The drawing under review shows one solid part. Ordinate dimensions are in mm from its lowest x, y, z. Give positions to 0.01 mm unless a question says otherwise; leave off trailing zeros. Write each loop counter-clockwise with the first axis right and the second up, starting at its lowest first coordinate (ties: lowest second). Pieces come first, ordered by that corner, then holes. Notation, with made-up numbers: (86, 12.25) -> (141, 12.25) arc R13 cw to (141, 26.25) -> close; hole circle Ø2 at (-22, 76.5). An arc over 180 degrees is marked (long way). Put each result on its own line as item: value. Start each with the question number.
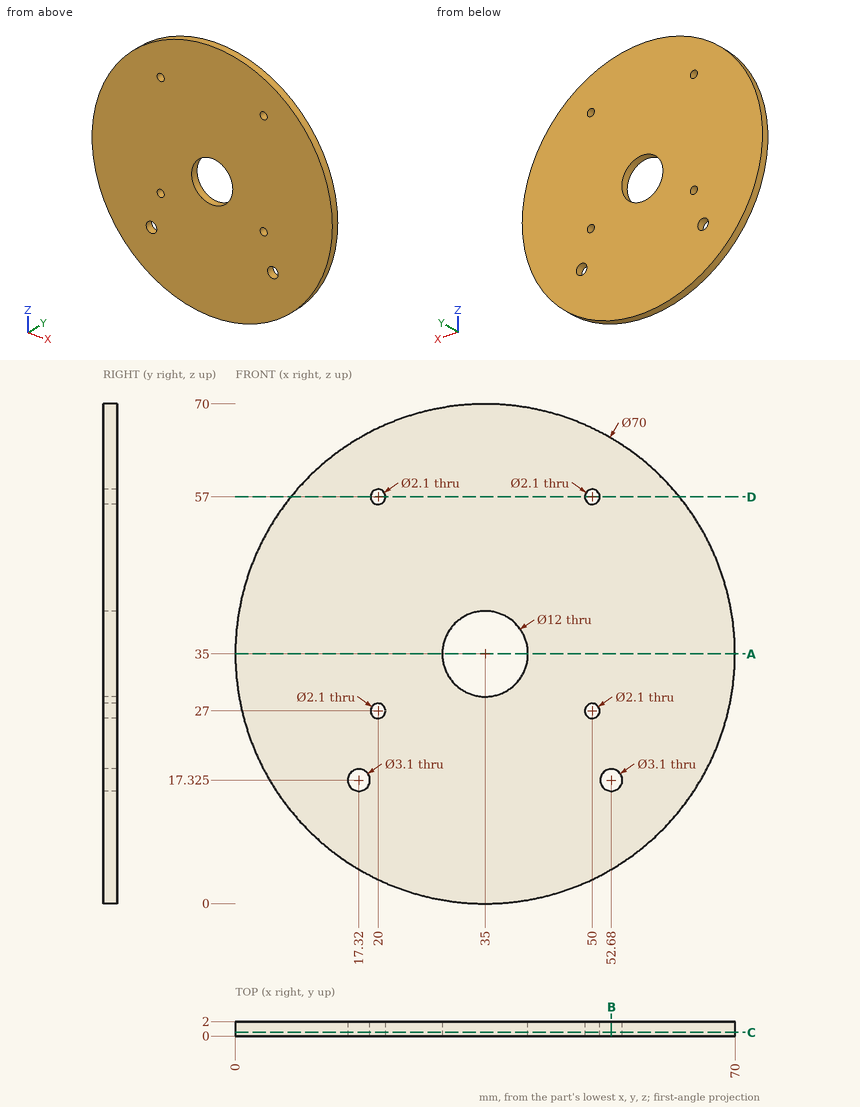
Q1. Take a section at A-A on z = 35. Give the boundary of the cut face in (x, y).
Q2. Take a section at D-D on z = 57. Give the boundary of the cut face in (x, y).
Q3. Take a section at B-B on x = 52.68. Give the boundary of the cut face in (y, z) (1 decimal).
Q4. To check wall thickness, follow probe 1 along Z at (x, y) = (35, 1.2); probe 2 along Z at (x, y) = (50, 1.05); probe 3 along X at (y, z) = (1.6, 30.5). State the ranges of each line that lie inside material, in increasing order. Write a range as from..to.
Q5. For pin 1 (1 mm diameter, centred on y = 1.5, z = 28, fed in from +X); pin 2 (1 mm diameter, centred on x = 34, y = 1.5, fed in from -Z), all flat-tipped, find the tip position at first contact; note any pin that passes through.
Q6. Take a section at C-C on y = 0.5. State how many separate pieces and enclosed holes the cut face has, then the cut area to 3 significant figures.
Result:
1. outline: (0, 0) -> (29, 0) -> (29, 2) -> (0, 2) -> close; (41, 0) -> (70, 0) -> (70, 2) -> (41, 2) -> close
2. outline: (7.78, 0) -> (18.95, 0) -> (18.95, 2) -> (7.78, 2) -> close; (21.05, 0) -> (48.95, 0) -> (48.95, 2) -> (21.05, 2) -> close; (51.05, 0) -> (62.22, 0) -> (62.22, 2) -> (51.05, 2) -> close
3. outline: (0, 4.8) -> (2, 4.8) -> (2, 15.8) -> (0, 15.8) -> close; (0, 18.9) -> (2, 18.9) -> (2, 65.2) -> (0, 65.2) -> close
4. probe 1: z = 0..29, 41..70
4. probe 2: z = 3.38..25.95, 28.05..55.95, 58.05..66.62
4. probe 3: x = 0.29..31.03, 38.97..69.71
5. pin 1: stops at x = 69.39
5. pin 2: stops at z = 0
6. separate pieces: 1
6. enclosed holes: 7
6. area: 3,710 mm^2
